Geometry: final body of the model. Coordinates: model frame, mm. A direction names the side the tool comes from. Give positions to 0.01 mm unless a question says otherwise; leave off trailing zeros. Loops run counter-clockwise (first coordinate to the right, second up) from the corner with the lowest first, then second, coordinate; pieces in that order, holes last. Notation, with made-up numbers: M 62,23.25 L 80,23.25 A21 ccw 80,31.25 Z; hole C 75,67 d5. An arc over 180 degrees is marked long. Put each result on its own line as item: value.
```python
from build123d import *

# Parameters (mm, degrees)
F0_W           = 80
F0_H           = 70
F0_W_2         = 65
F0_H_2         = 57
F1_DEPTH       = 5
F2_R           = 2
F5_D           = 2.8
F5_DEPTH       = 5
F5_START       = 0.213943
F5_CBORE_D     = 5.8
F5_CBORE_DEPTH = 2.5
F5_TIP         = 0.8412048666
F7_W           = 65
F7_H           = 57
F7_W_2         = 57
F7_H_2         = 49
F8_DEPTH       = 2.3


with BuildPart() as f1:
    # F0 (on Front) → F1 (new body)
    with BuildSketch(Plane.XZ):
        Rectangle(F0_W, F0_H)
        Rectangle(F0_W_2, F0_H_2, mode=Mode.SUBTRACT)
    extrude(amount=F1_DEPTH)

    # F2
    f2_edges = [f1.edges().sort_by_distance(p)[0] for p in [
        (0, 0, 35),
        (-40, 0, 0),
        (-40, -2.5, 35),
        (0, 0, -35),
        (-40, -2.5, -35),
        (40, 0, 0),
        (40, -2.5, -35),
        (40, -2.5, 35),
    ]]
    fillet(f2_edges, radius=F2_R)

    # F5
    # its depths count from where the whole tool has entered the part; down to there all is cleared
    with Locations(Plane(origin=(0, 0, 0), x_dir=(-1, 0, 0), z_dir=(0, 1, 0)).offset(-F5_START)):
        with Locations((-36, -31), (-36, 31), (36, 31), (36, -31)):
            CounterBoreHole(F5_D / 2, F5_CBORE_D / 2, F5_CBORE_DEPTH, depth=F5_DEPTH)
            with Locations((0, 0, -(F5_DEPTH + F5_TIP / 2))):  # 118° drill point
                Cone(0, F5_D / 2, F5_TIP, mode=Mode.SUBTRACT)

    # F7 (on offset) → F8 (join)
    with BuildSketch(Plane.XZ.offset(5)):
        Rectangle(F7_W, F7_H)
        Rectangle(F7_W_2, F7_H_2, mode=Mode.SUBTRACT)
    extrude(amount=-F8_DEPTH)


solid = f1.part
```
Item 1: Section D-D on x = 36. Output: boundary loops of the cut face in (y, z), then the cut area to 3 significant figures.
Output values:
outline: M -5,-35 L -2,-35 A2 ccw -0.21,-33.9 L -2.71,-33.9 L -2.71,-32.4 L -5,-32.4 Z; M -5,-29.6 L -2.71,-29.6 L -2.71,-28.1 L 0,-28.1 L 0,28.1 L -2.71,28.1 L -2.71,29.6 L -5,29.6 Z; M -5,32.4 L -2.71,32.4 L -2.71,33.9 L -0.21,33.9 A2 ccw -2,35 L -5,35 Z
area: 304 mm²
Item 2: Set-up query: faces 1 (the flat face through (28.5, -4, 0)), 2 (the flat face through (-12, -5, 26)), 3 (the flat face through (-32.5, -1, 0)). Return all of +Z, -Z, +X, -X, +Y, -Y with unobstructed straight access to the full face (end or side cutting, diameter ignored); none if empty.
Output values:
face 1: +Y, -Y
face 2: +Z, -Z, +X, -X, -Y
face 3: +Y
Item 3: Pin query (flat end, axial travel): pin 1 Ø4.5 at (x, z) = (-36, -31) entering from +Y; pin 2 Ø6.5 at (x, z) = (-35.5, -31.5) entering from +Y; pin 3 Ø0.8 at (y, z) = (-1.5, -0.5) entering from +X. Return the tip coordinate at first contact, or that it passes through.
Output values:
pin 1: y = -2.71
pin 2: y = 0
pin 3: x = 40
Item 4: Line query: probe 1 along Z at (x, y) = (-36, -3.35); probe 2 along X at (y, z) = (-4.4, -1); probe 3 along Z at (x, y) = (-20, -3.6). Output: solid intervals per line, ascending. Write a range as [from, to].
Output values:
probe 1: [-35, -32.4], [-29.6, 29.6], [32.4, 35]
probe 2: [-40, -28.5], [28.5, 40]
probe 3: [-35, -24.5], [24.5, 35]
Item 5: Section B-B on z = 7. Output: boundary loops of the cut face in (x, y).
Output values:
outline: M -40,-5 L -28.5,-5 L -28.5,-2.7 L -32.5,-2.7 L -32.5,0 L -38,0 A2 ccw -40,-2 Z; M 28.5,-5 L 40,-5 L 40,-2 A2 ccw 38,0 L 32.5,0 L 32.5,-2.7 L 28.5,-2.7 Z
Item 6: Mould query, pull axis X, two halves, no side actions, for faces 4 (the cylindrical face through (-35.25, -3.87, -29.82)), 5 (the flat face through (-1, -3, -35)), 6 (the cylindrical face through (39.4, -3.52, -34.43)), 7 (the cylindrical face through (33.234, -1.338, -30.129)). Classes: pulls with the +X half, pulls with the -X half, needs draft (parallel to the pull), parting line crosses it, or undercut.
Output values:
face 4: undercut
face 5: needs draft
face 6: pulls with the +X half
face 7: undercut
Item 7: Section C-C on x = -24. Output: boundary loops of the cut face in (y, z).
Output values:
outline: M -5,-35 L -2,-35 A2 ccw 0,-33 L 0,-28.5 L -2.7,-28.5 L -2.7,-24.5 L -5,-24.5 Z; M -5,24.5 L -2.7,24.5 L -2.7,28.5 L 0,28.5 L 0,33 A2 ccw -2,35 L -5,35 Z
Item 8: Section A-A on y = -4. Output: boundary loops of the cut face in (x, z).
Output values:
outline: M -40,-33 A2 ccw -38,-35 L 38,-35 A2 ccw 40,-33 L 40,33 A2 ccw 38,35 L -38,35 A2 ccw -40,33 Z; hole C -36,-31 d2.8; hole C -36,31 d2.8; hole M -28.5,-24.5 L 28.5,-24.5 L 28.5,24.5 L -28.5,24.5 Z; hole C 36,-31 d2.8; hole C 36,31 d2.8
